```python
from build123d import *


with BuildPart() as part:
    # 草图1 → 旋转1 (revolve)
    with BuildSketch(Plane.XY, mode=Mode.PRIVATE) as revolve_1_sk:
        Polygon((0, 5), (0, 9), (18, 9), (25, 6), (25, 0), (0, 0), (-12, 0), (-12, 5), align=None)
    revolve(revolve_1_sk.sketch.rotate(Axis((25, 0, 0), (-1, 0, 0)), 90), axis=Axis((25, 0, 0), (-1, 0, 0)))

    # 切除-拉伸1 cone 1 section (through the dimple's axis) → 切除-拉伸1 (revolve, cut)
    with BuildSketch(Plane(origin=(25, 0, 0), x_dir=(0, 0, -1), z_dir=(0, 1, 0))):
        Polygon((0, 0), (0.6, 0), (0, 0.6), align=None)
    revolve(axis=Axis((25, 0, 0), (-1, 0, 0)), mode=Mode.SUBTRACT)


solid = part.part
```
Work out the finished part from the listing and answer in its coordinate system (mm). A direction names the side the tool comes from. Give positions to 0.01 mm unless a question says otherwise; leave off trailing zeros. Write each loop counter-clockwise with the first axis right and the second up, starting at its lowest first coordinate (ties: lowest second). Pieces come first, ordered by that corner, then holes. Notation, with made-up numbers: (35.25, 29.5) -> (86.25, 29.5) arc R12 cw to (86.25, 43.5) -> close; hole circle Ø4 at (72, -27.75). An arc over 180 degrees is marked (long way). Write item = value, one per line.
Q1. Flat-ended cylindrical pins translate along their axes: pin 1 Ø1.5 at (x, y) = (-5, -1.5) entering from -Z; pin 2 Ø4 at (x, z) = (18, 5.5) entering from -Y; pin 3 Ø4 at (x, y) = (5.5, -6) entering from -Z. Find the tip coordinate at first contact, or state that the pin passes through.
Computed values:
pin_1 = -4.94
pin_2 = -8.29
pin_3 = -8.06
Q2. Consider line 1 along X through (y, z) = (-5, -3.25); line 2 along Y through (x, z) = (10, -4.5); line 3 along X through (y, z) = (-7, -4.75). Determine where each line is inside the solid, lowest interval first.
Computed values:
line_1 = 0 to 25
line_2 = -7.79 to 7.79
line_3 = 0 to 19.26
Q3. Section A-A on x = 1.5 is taken. Determine the outline of the cut face in (y, z), and give its area (3 significant figures).
Computed values:
outline = circle Ø18 at (0, 0)
area = 254 mm^2
Q4. A tool of negligible diameter and unlimited length cuts with its end or side. For faces 1 (the flat face through (0, 4, 4)), 2 (the flat face through (25, 0, -1)), from which of +Z, -Z, +X, -X, +Y, -Y can it reach the whole face along a straight path? Write none if from no direction.
Computed values:
face_1 = -X
face_2 = +Z, -Z, +X, +Y, -Y
